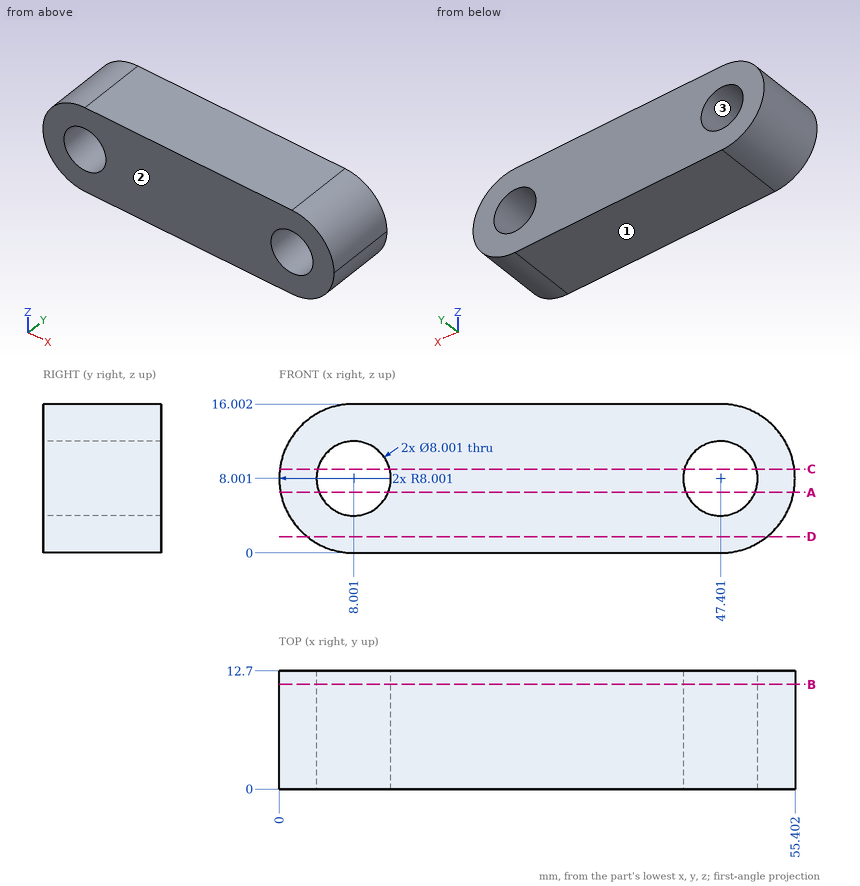
Can you work these out from the drawing? Everything is in mm from the part's minimum corner. Round coordinates to 2 decimals unless told otherwise and drop trailing zeros. Write each loop counter-clockwise with the first axis right and the second up, starting at its lowest first coordinate (ties: lowest second). Pieces come first, ordered by that corner, then holes. Notation, with made-up numbers: (36, -5.75) - (76, -5.75) arc R30 cw to (76, 22.25) - close; hole circle Ø4 at (4.5, 43). An arc over 180 degrees is marked (long way). Use a Markdown table: item, result.
Q1. I want a section at A-A (z = 6.5). List the corners of the cut face in (x, y) for me, plus the area to 3 significant figures.
Output values:
| item | result |
|---|---|
| outline | (0.14, 0) - (4.29, 0) - (4.29, 12.7) - (0.14, 12.7) - close; (11.71, 0) - (43.69, 0) - (43.69, 12.7) - (11.71, 12.7) - close; (51.11, 0) - (55.26, 0) - (55.26, 12.7) - (51.11, 12.7) - close |
| area | 512 mm2 |
Q2. Please list where these lines run through material, in increasing order: L1, parallel to X at y = 1.75, z = 6; L2, parallel to X at y = 4, z = 6.5; L3, parallel to Z at x = 44.5, y = 3.5.
Output values:
| item | result |
|---|---|
| L1 | 0.25 to 4.54, 11.47 to 43.94, 50.87 to 55.15 |
| L2 | 0.14 to 4.29, 11.71 to 43.69, 51.11 to 55.26 |
| L3 | 0 to 5.25, 10.76 to 16 |
Q3. Thinking about a two-plate mould opening in Z: for the marked faces 1, 2 and 3, which applies, released by +Z, released by -Z, zero draft, split by the parting line, or undercut?
Output values:
| item | result |
|---|---|
| face 1 | released by -Z |
| face 2 | zero draft |
| face 3 | undercut |
Q4. I want a section at C-C (z = 9). List the corners of the cut face in (x, y) for me, plus the area to 3 significant figures.
Output values:
| item | result |
|---|---|
| outline | (0.06, 0) - (4.13, 0) - (4.13, 12.7) - (0.06, 12.7) - close; (11.87, 0) - (43.53, 0) - (43.53, 12.7) - (11.87, 12.7) - close; (51.27, 0) - (55.34, 0) - (55.34, 12.7) - (51.27, 12.7) - close |
| area | 505 mm2 |
Q5. I want a section at B-B (y = 11.25). List the corners of the cut face in (x, z) for me.
Output values:
| item | result |
|---|---|
| outline | (8, 0) - (47.4, 0) arc R8 ccw to (55.4, 8) arc R8 ccw to (47.4, 16) - (8, 16) arc R8 ccw to start; hole circle Ø8 at (8, 8); hole circle Ø8 at (47.4, 8) |
Q6. I want a section at D-D (z = 1.75). List the corners of the cut face in (x, y) for me.
Output values:
| item | result |
|---|---|
| outline | (3.01, 0) - (52.4, 0) - (52.4, 12.7) - (3.01, 12.7) - close |
Q7. For pin 1 (5 mm diameter, centred on y = 11, z = 13.5, fed in from -X); pin 2 (2 mm diameter, centred on y = 7, z = 3, fed in from -X); pin 3 (5 mm diameter, centred on y = 10, z = 4, fed in from +X), each with a flat end and sliding along its axis, tell me the tip position at first contact or that it passes through.
Output values:
| item | result |
|---|---|
| pin 1 | x = 0.58 |
| pin 2 | x = 1.07 |
| pin 3 | x = 55.26 |
